from build123d import *

# Parameters (mm, degrees)
SKETCH1_R               = 8
SKETCH1_R_2             = 7
BOSS_EXTRUDE1_DEPTH     = 15
SKETCH2_R               = 9
SKETCH2_R_2             = 8
BOSS_EXTRUDE2_DEPTH     = 120
SKETCH3_R               = 8
SKETCH3_R_2             = 7
CUT_EXTRUDE1_DEPTH      = 5
CUT_EXTRUDE2_DEPTH      = 31
CUT_EXTRUDE2_DEPTH_BACK = 31
SKETCH4_W               = 18
SKETCH4_H               = 40.940584593
CUT_EXTRUDE3_DEPTH      = 31
CUT_EXTRUDE3_DEPTH_BACK = 31
SKETCH5_W               = 18
SKETCH5_H               = 23.079337433


with BuildPart() as part:
    # Sketch1 → Boss-Extrude1 (new body)
    with BuildSketch(Plane(origin=(0, 0, 0), x_dir=(1, 0, 0), z_dir=(0, 1, 0))):
        with Locations(Location((0, 0, 0), (0, 0, 270))):
            Circle(SKETCH1_R)
        with Locations(Location((0, 0, 0), (0, 0, 270))):
            Circle(SKETCH1_R_2, mode=Mode.SUBTRACT)
    extrude(amount=BOSS_EXTRUDE1_DEPTH)

    # Sketch2 → Boss-Extrude2 (add)
    with BuildSketch(Plane(origin=(0, 10, 0), x_dir=(1, 0, 0), z_dir=(0, 1, 0))):
        with Locations(Location((0, 0, 0), (0, 0, 270))):
            Circle(SKETCH2_R)
        with Locations(Location((0, 0, 0), (0, 0, 270))):
            Circle(SKETCH2_R_2, mode=Mode.SUBTRACT)
    extrude(amount=BOSS_EXTRUDE2_DEPTH)

    # Sketch3 → Cut-Extrude1 (cut)
    with BuildSketch(Plane(origin=(0, 0, 0), x_dir=(1, 0, 0), z_dir=(0, 1, 0))):
        with Locations(Location((0, 0, 0), (0, 0, 270))):
            Circle(SKETCH3_R)
        with Locations(Location((0, 0, 0), (0, 0, 270))):
            Circle(SKETCH3_R_2, mode=Mode.SUBTRACT)
    extrude(amount=CUT_EXTRUDE1_DEPTH, mode=Mode.SUBTRACT)

    # Sketch4 → Cut-Extrude2 (cut, two sides: drawn at the far end of the back side and taken through both)
    with BuildSketch(Plane.XY.offset(-CUT_EXTRUDE2_DEPTH_BACK)):
        with Locations((0, 109.529707704)):
            Rectangle(SKETCH4_W, SKETCH4_H)
    extrude(amount=CUT_EXTRUDE2_DEPTH + CUT_EXTRUDE2_DEPTH_BACK, mode=Mode.SUBTRACT)

    # Sketch5 → Cut-Extrude3 (cut, two sides: drawn at the far end of the back side and taken through both)
    with BuildSketch(Plane.XY.offset(-CUT_EXTRUDE3_DEPTH_BACK)):
        with Locations((0, 77.51974669)):
            Rectangle(SKETCH5_W, SKETCH5_H)
    extrude(amount=CUT_EXTRUDE3_DEPTH + CUT_EXTRUDE3_DEPTH_BACK, mode=Mode.SUBTRACT)


solid = part.part
Work out the finished part from the listing and answer in its coordinate system (mm). A direction names the side the tool comes from. Coordinates: 2 decimals unless noted, no trailing zeros. Order: outer loops, then holes, each group sorted by start corner. A loop starts at its lowest first (then second) coordinate and runs counter-clockwise, first axis right, second up. Notation, with made-up numbers: (-8, 43) - (50, 43) arc R14 ccw to (50, 49) - close; hole circle Ø3 at (52.25, 2.25). An arc over 180 degrees is marked (long way). Put each result on its own line as item: value. Start each with the question number.
1) Find the intervals of material crossed by line 1 (X direction, y = 36, z = 0); line 2 (X direction, y = 12.5, z = 0); line 3 (Y direction, x = -6, z = 3.75), in increasing order. Write a range as from..to.
2) Find section B-B (z = 0). Give the vertices of the cut face in (x, y).
3) For faces 5 (the cylindrical face through (2.703, 37.598, 8.584)), 6 (the cylindrical face through (-7.81, 40.13, -1.73)), determine the directions among +Z, -Z, +X, -X, +Y, -Y from which every point of the face is accessible in a straight line to the end or side of a thin tool.
4) For a pull along X with two mould halves and no side action, classify faces 1 (the cylindrical face through (-6.834, 9.93, -1.517)), 2 (the cylindrical face through (-7.81, 7.46, -1.73)), 3 (the flat face through (-6, 5, 4)), 4 (the flat face through (-6, 15, 4)) as released by +X, released by -X, zero draft, split by the parting line, or undercut.
5) Flat-ended cylindrical pins translate along their axes: pin 1 (5 mm diameter, centred on x = 3.5, z = 1.5, fed in from +Y); pin 2 (3 mm diameter, centred on y = 56, z = -5, fed in from +X); pin 3 (2 mm diameter, centred on y = 44, z = 7, fed in from +X). Find the tip coordinate at first contact, or state that the pin passes through.
6) Find section C-C (y = 27). Give the vertices of the cut face in (x, z), plus the area to 3 significant figures.
7) Find section A-A (x = 0). Give the vertices of the cut face in (y, z).
Results list:
1. line 1: x = -9..-8, 8..9
1. line 2: x = -9..-7, 7..9
1. line 3: y = 5..15
2. outline: (-9, 10) - (-8, 10) - (-8, 5) - (-7, 5) - (-7, 15) - (-8, 15) - (-8, 65.98) - (-9, 65.98) - close; (7, 5) - (8, 5) - (8, 10) - (9, 10) - (9, 65.98) - (8, 65.98) - (8, 15) - (7, 15) - close
3. face 5: +Y, -Y
3. face 6: +Y
4. face 1: undercut
4. face 2: split by the parting line
4. face 3: zero draft
4. face 4: undercut
5. pin 1: passes through
5. pin 2: stops at x = 8.29
5. pin 3: stops at x = 6.71
6. outline: circle Ø18 at (0, 0); hole circle Ø16 at (0, 0)
6. area: 53.4 mm^2
7. outline: (5, -8) - (10, -8) - (10, -9) - (65.98, -9) - (65.98, -8) - (15, -8) - (15, -7) - (5, -7) - close; (5, 7) - (15, 7) - (15, 8) - (65.98, 8) - (65.98, 9) - (10, 9) - (10, 8) - (5, 8) - close
